from build123d import *

# Parameters (mm, degrees)
SKETCH1_R               = 4
BOSS_EXTRUDE1_DEPTH     = 123.825
CUT_EXTRUDE1_DEPTH      = 124.954147268
CUT_EXTRUDE1_DEPTH_BACK = 124.954147268
SKETCH3_W               = 19.05
SKETCH3_H               = 1.65
SKETCH3_W_2             = 40.878125


with BuildPart() as part:
    # Sketch1 → Boss-Extrude1 (new, symmetric)
    with BuildSketch(Plane(origin=(0, 0, 0), x_dir=(0, 0, -1), z_dir=(1, 0, 0))):
        Circle(SKETCH1_R)
    extrude(amount=BOSS_EXTRUDE1_DEPTH, both=True)

    # Sketch3 → Cut-Extrude1 (cut, two sides: drawn at the far end of the back side and taken through both)
    with BuildSketch(Plane.XY.offset(-CUT_EXTRUDE1_DEPTH_BACK)):
        with Locations((-114.3, 3.175)):
            Rectangle(SKETCH3_W, SKETCH3_H)
        with Locations((103.3859375, 3.175)):
            Rectangle(SKETCH3_W_2, SKETCH3_H)
    extrude(amount=CUT_EXTRUDE1_DEPTH + CUT_EXTRUDE1_DEPTH_BACK, mode=Mode.SUBTRACT)


solid = part.part
Source: CAD feature listing. Evaluate the final solid. Frame: model axes, mm. A direction names the side the tool comes from. Round coordinates to 2 decimals unless told otherwise and drop trailing zeros. Loops run counter-clockwise (first coordinate to the right, second up) from the corner with the lowest first, then second, coordinate; pieces in that order, holes last.
Q1. Access query for faces 1 (the face through (-114, 2.35, 0)), 2 (the face through (1.734, -3.905, 0.867)), 3 (the face through (103, 2.35, 0)). Directions: +Z, -Z, +X, -X, +Y, -Y. A direction counts if a zero-diameter tool reaches every point of the face in a straight line with its end or side. Return the directions, or none.
Q2. Ray query, line 1 (Y direction, x = 101, z = -0.5); line 2 (Z direction, x = 105, y = -0.25); line 3 (Z direction, x = -43.5, y = 1.5). Return the intervals inside material, ascending.
Q3. First-contact query: P1, Ø2, axis at x = -85, z = -2, coming from the -Y side; P2, Ø1.9, axis at x = -113, z = -0.5, coming from the +Y side; P3, Ø3, axis at x = 96.5, y = -3, coming from the -Z side. Flat tips, straight axial feed; report the tip coordinate or a pass-through.
Q4. Section A-A, the plane z = -2. Return loops of the section in (x, y) (3 decimals).
Q5. Section B-B, the plane x = 93.5. Return loops of the section in (y, z).
Q6. Section C-C, the plane x = 46. Return loops of the section in (y, z), plus the area to 3 significant figures.
Solutions:
1. face 1: +Z, -Z, -X, +Y
1. face 2: +X, -X
1. face 3: +Z, -Z, +X, +Y
2. line 1: y = -3.97 to 2.35
2. line 2: z = -3.99 to 3.99
2. line 3: z = -3.71 to 3.71
3. P1: stops at y = -3.87
3. P2: stops at y = 2.35
3. P3: stops at z = -3.71
4. outline: (-123.825, -3.464) - (123.825, -3.464) - (123.825, 2.35) - (82.947, 2.35) - (82.947, 3.464) - (-104.775, 3.464) - (-104.775, 2.35) - (-123.825, 2.35) - close
5. outline: (2.35, -3.24) - (2.35, 3.24) arc R4 ccw (long way) to start
6. outline: circle Ø8 at (0, 0)
6. area: 50.3 mm2
